```python
from build123d import *

# Parameters (mm, degrees)
F0_W     = 5.08
F0_H     = 6.35
F1_DEPTH = 2.9718
F2_W     = 3.048
F2_H     = 14.9098
F2_H_2   = 44.704
F2_R     = 1.651
F3_DEPTH = 25.4


with BuildPart() as f1:
    # F0 (on Top) → F1 (new body)
    with BuildSketch(Plane.XY):
        with Locations((194.818, 37.465)):
            Rectangle(F0_W, F0_H)
        with Locations((194.818, 13.335)):
            Rectangle(F0_W, F0_H)
        Polygon((0, 50.8), (0, 0), (192.278, 0), (192.278, 10.16), (192.278, 16.51), (192.278, 34.29), (192.278, 40.64), (192.278, 50.8), align=None)
    extrude(amount=F1_DEPTH)

    # F2 (on face) → F3 (intersect)
    with BuildSketch(Plane.XY.offset(2.9718)):
        Polygon((0, 50.8), (0, 41.656), (3.048, 41.656), (3.048, 39.116), (8.128, 39.116), (8.128, 41.148), (11.938, 41.148), (11.938, 39.116), (14.986, 39.116), (14.986, 35.814), (11.938, 35.814), (11.938, 33.782), (8.128, 33.782), (8.128, 35.814), (3.048, 35.814), (3.048, 33.274), (0, 33.274), (0, 17.526), (3.048, 17.526), (3.048, 14.986), (8.128, 14.986), (8.128, 17.018), (11.938, 17.018), (11.938, 14.986), (14.986, 14.986), (14.986, 11.684), (11.938, 11.684), (11.938, 9.652), (8.128, 9.652), (8.128, 11.684), (3.048, 11.684), (3.048, 9.144), (0, 9.144), (0, 0), (45.72, 0), (45.72, 14.9098), (48.768, 14.9098), (48.768, 0), (70.104, 0), (70.104, 14.9098), (73.152, 14.9098), (73.152, 0), (82.296, 0), (82.296, 14.9098), (85.344, 14.9098), (85.344, 0), (94.488, 0), (94.488, 14.9098), (97.536, 14.9098), (97.536, 0), (106.68, 0), (106.68, 14.9098), (109.728, 14.9098), (109.728, 0), (131.064, 0), (131.064, 14.9098), (134.112, 14.9098), (134.112, 0), (143.256, 0), (143.256, 14.9098), (146.304, 14.9098), (146.304, 0), (192.278, 0), (192.278, 10.16), (197.358, 10.16), (197.358, 16.51), (192.278, 16.51), (192.278, 34.29), (197.358, 34.29), (197.358, 40.64), (192.278, 40.64), (192.278, 50.8), (146.304, 50.8), (146.304, 35.8902), (143.256, 35.8902), (143.256, 50.8), (134.112, 50.8), (134.112, 35.8902), (131.064, 35.8902), (131.064, 50.8), (121.92, 50.8), (121.92, 35.9664), (118.872, 35.9664), (118.872, 50.8), (109.728, 50.8), (109.728, 35.8902), (106.68, 35.8902), (106.68, 50.8), (97.536, 50.8), (97.536, 35.8902), (94.488, 35.8902), (94.488, 50.8), (85.344, 50.8), (85.344, 35.8902), (82.296, 35.8902), (82.296, 50.8), (73.152, 50.8), (73.152, 35.8902), (70.104, 35.8902), (70.104, 50.8), (60.96, 50.8), (60.96, 35.9664), (57.912, 35.9664), (57.912, 50.8), (48.768, 50.8), (48.768, 35.8902), (45.72, 35.8902), (45.72, 50.8), align=None)
        with Locations((59.436, 7.5311)):
            Rectangle(F2_W, F2_H, mode=Mode.SUBTRACT)
        with Locations((41.148, 25.4)):
            Rectangle(F2_W, F2_H_2, mode=Mode.SUBTRACT)
        with Locations((47.244, 25.3873)):
            Rectangle(F2_W, F2_H, mode=Mode.SUBTRACT)
        with Locations((65.532, 25.4)):
            Rectangle(F2_W, F2_H_2, mode=Mode.SUBTRACT)
        with Locations((71.628, 25.3873)):
            Rectangle(F2_W, F2_H, mode=Mode.SUBTRACT)
        with Locations((77.724, 25.4)):
            Rectangle(F2_W, F2_H_2, mode=Mode.SUBTRACT)
        with Locations((83.82, 25.3873)):
            Rectangle(F2_W, F2_H, mode=Mode.SUBTRACT)
        with Locations((89.916, 25.4)):
            Rectangle(F2_W, F2_H_2, mode=Mode.SUBTRACT)
        with Locations((96.012, 25.3873)):
            Rectangle(F2_W, F2_H, mode=Mode.SUBTRACT)
        with Locations((120.396, 7.5311)):
            Rectangle(F2_W, F2_H, mode=Mode.SUBTRACT)
        with Locations((102.108, 25.4)):
            Rectangle(F2_W, F2_H_2, mode=Mode.SUBTRACT)
        with Locations((108.204, 25.3873)):
            Rectangle(F2_W, F2_H, mode=Mode.SUBTRACT)
        with Locations((114.3, 25.4)):
            Rectangle(F2_W, F2_H_2, mode=Mode.SUBTRACT)
        with Locations((132.588, 25.3873)):
            Rectangle(F2_W, F2_H, mode=Mode.SUBTRACT)
        with Locations((138.684, 25.4)):
            Rectangle(F2_W, F2_H_2, mode=Mode.SUBTRACT)
        with Locations((144.78, 25.3873)):
            Rectangle(F2_W, F2_H, mode=Mode.SUBTRACT)
        with Locations((193.7639, 13.335)):
            Circle(F2_R, mode=Mode.SUBTRACT)
        with Locations((150.876, 25.4)):
            Rectangle(F2_W, F2_H_2, mode=Mode.SUBTRACT)
        Polygon((54.864, 3.1242), (51.816, 3.1242), (51.816, 17.9324), (51.816, 32.8422), (51.816, 47.8282), (54.864, 47.8282), align=None, mode=Mode.SUBTRACT)
        with Locations((59.436, 25.4635)):
            Rectangle(F2_W, F2_H, mode=Mode.SUBTRACT)
        with Locations((120.396, 25.4635)):
            Rectangle(F2_W, F2_H, mode=Mode.SUBTRACT)
        with Locations((126.492, 25.4762)):
            Rectangle(F2_W, F2_H_2, mode=Mode.SUBTRACT)
        with Locations((193.7639, 37.465)):
            Circle(F2_R, mode=Mode.SUBTRACT)
    extrude(amount=-F3_DEPTH, mode=Mode.INTERSECT)


solid = f1.part
```
Check sheet for the modelled part. Datum: model origin and axes. Units: mm. Coordinates: 2 decimals unless noted, no trailing zeros. Use a Markdown table: item, result.
1. Sectioned sample at A-A (y = 29.5). Give the number of separate pieces and of enclosed holes in the cut face, plus the area to 3 significant figures.
Reported:
| item | result |
|---|---|
| separate pieces | 20 |
| enclosed holes | 0 |
| area | 399 mm2 |
2. Release check for a two-part mould opening along Y. For faces 1 (the cylindrical face through (195.34, 37.96, 1.51)), 2 (the flat face through (75, 26, 0)), 3 (the cylindrical face through (195.34, 13.83, 1.51)) record: pulls with the +Y half, pulls with the -Y half, needs draft (parallel to the pull), parting line crosses it, or undercut.
Reported:
| item | result |
|---|---|
| face 1 | undercut |
| face 2 | needs draft |
| face 3 | undercut |
3. Scan lines: line 1 along Y through (x, z) = (90.5, 0.5); line 2 along Y through (x, z) = (85, 2). Record each from-to range of solid material in increasing order.
Reported:
| item | result |
|---|---|
| line 1 | y = 0 to 3.05, 47.75 to 50.8 |
| line 2 | y = 14.91 to 17.93, 32.84 to 35.89 |
4. Go/stop test with flat-tipped pins: pin 1 Ø1.5 at (y, z) = (41.5, 1) entering from +X; pin 2 Ø0.9 at (x, z) = (46.5, 1) entering from +Y. Record where each tip stops, or that it passes through.
Reported:
| item | result |
|---|---|
| pin 1 | stops at x = 192.28 |
| pin 2 | stops at y = 35.89 |
